```python
from build123d import *

# Parameters (mm, degrees)
F1_DEPTH = 40
F3_D     = 10
F3_DEPTH = 38.5
F3_TIP   = 3.0043030951
F4_DEPTH = 2
F5_R     = 1


with BuildPart() as f1:
    # F0 (on Top) → F1 (new body)
    with BuildSketch(Plane.XY):
        with BuildLine():
            ThreePointArc((0, -5), (-5, 0), (0, 5))
            Line((0, 5), (0, 9))
            ThreePointArc((0, 9), (-5.0605227038, 7.442520404), (-8.3695652174, 3.3091355475))
            ThreePointArc((-8.3695652174, 3.3091355475), (-8, 0), (-8.3695652174, -3.3091355475))
            ThreePointArc((-8.3695652174, -3.3091355475), (-5.0605227038, -7.442520404), (0, -9))
            Line((0, -9), (0, -5))
        make_face()
        with BuildLine():
            ThreePointArc((-8.3695652174, 3.3091355475), (-5.0605227038, 7.442520404), (0, 9))
            Line((0, 9), (-11, 9))
            ThreePointArc((-11, 9), (-9.3841453176, 6.2935285229), (-8.3695652174, 3.3091355475))
        make_face()
        with BuildLine():
            Line((-11, -9), (0, -9))
            ThreePointArc((0, -9), (-5.0605227038, -7.442520404), (-8.3695652174, -3.3091355475))
            ThreePointArc((-8.3695652174, -3.3091355475), (-9.3841453176, -6.2935285229), (-11, -9))
        make_face()
        with BuildLine():
            ThreePointArc((0, 5), (3.5355339059, 3.5355339059), (5, 0))
            ThreePointArc((5, 0), (3.5355339059, -3.5355339059), (0, -5))
            Line((0, -5), (0, -9))
            ThreePointArc((0, -9), (6.3639610307, -6.3639610307), (9, 0))
            ThreePointArc((9, 0), (6.3639610307, 6.3639610307), (0, 9))
            Line((0, 9), (0, 5))
        make_face()
        with BuildLine():
            Line((0, -5), (0, 5))
            ThreePointArc((0, 5), (-5, 0), (0, -5))
        make_face()
        with BuildLine():
            ThreePointArc((0, -5), (3.5355339059, -3.5355339059), (5, 0))
            ThreePointArc((5, 0), (3.5355339059, 3.5355339059), (0, 5))
            Line((0, 5), (0, -5))
        make_face()
    extrude(amount=F1_DEPTH)

    # F3
    with Locations(Plane(origin=(0, 0, 0), x_dir=(1, 0, 0), z_dir=(0, 0, -1))):
        with Locations((0, 0)):
            Hole(F3_D / 2, depth=F3_DEPTH)
            with Locations((0, 0, -(F3_DEPTH + F3_TIP / 2))):  # 118° drill point
                Cone(0, F3_D / 2, F3_TIP, mode=Mode.SUBTRACT)

    # F4 (add): a face of the model
    f4_faces = [f1.faces().sort_by_distance(p)[0] for p in [
        (-5.5, 8.7309275191, 40),
    ]]
    extrude(f4_faces, amount=F4_DEPTH)

    # F5
    f5_edges = [f1.edges().sort_by_distance(p)[0] for p in [
        (-11, -9, 21),
        (-11, 9, 21),
    ]]
    fillet(f5_edges, radius=F5_R)


solid = f1.part
```
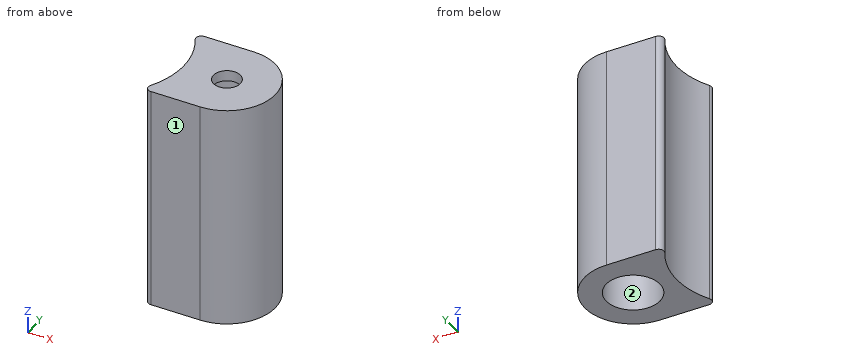
Source: CAD feature listing. Evaluate the final solid. Frame: model axes, mm. Face numbers are marked on the shaded views. A direction names the side the tool comes from. Give positions to 0.01 mm unless a question says otherwise; leave off trailing zeros. Write each loop counter-clockwise with the first axis right and the second up, starting at its lowest first coordinate (ties: lowest second). Pieces come first, ordered by that corner, then holes.
1. Access query for the marked faces 1 and 2. Directions: +Z, -Z, +X, -X, +Y, -Y. A direction counts if a zero-diameter tool reaches every point of the face in a straight line with its end or side. Return the directions, or none.
2. Section query A-A (y = 0). Return the cut outline in (x, z).
3. First-contact query: pin 1 (2 mm diameter, centred on y = -5.5, z = 20, fed in from +X); pin 2 (4 mm diameter, centred on y = 4, z = 37.5, fed in from +X); pin 3 (8 mm diameter, centred on x = 0, y = -0.5, fed in from -Z); pin 4 (4.5 mm diameter, centred on x = 0, y = 0, fed in from +Z). Flat tips, straight axial feed; report the tip coordinate or a pass-through.
4. Section query B-B (z = 12). Return the cut outline in (x, y).
5. Material intervals for line 1 along Y through (x, z) = (0, 30); line 2 along Y through (x, z) = (0, 40.9); line 3 along X through (y, z) = (0.75, 39.5), sorted ascending.
6. Section query C-C (y = 6.25). Return the cut outline in (x, z), then the cut area to 3 significant figures.
Output values:
1. face 1: +Z, -Z, +X, -X, -Y
1. face 2: -Z
2. outline: (-8, 0) - (-5, 0) - (-5, 38.5) - (-2.5, 40) - (-2.5, 42) - (-8, 42) - close; (2.5, 40) - (5, 38.5) - (5, 0) - (9, 0) - (9, 42) - (2.5, 42) - close
3. pin 1: stops at x = 7.79
3. pin 2: stops at x = 8.77
3. pin 3: stops at z = 38.8
3. pin 4: passes through
4. outline: (-10.01, -7.5) arc R1 ccw to (-9.14, -9) - (0, -9) arc R9 ccw to (0, 9) - (-9.14, 9) arc R1 ccw to (-10.01, 7.5) arc R15 cw to start; hole circle Ø10 at (0, 0)
5. line 1: y = -9 to -5, 5 to 9
5. line 2: y = -9 to -2.5, 2.5 to 9
5. line 3: x = -8.02 to -3.25, 3.25 to 8.97
6. outline: (-9.36, 0) - (6.48, 0) - (6.48, 42) - (-9.36, 42) - close
6. area: 665 mm2
